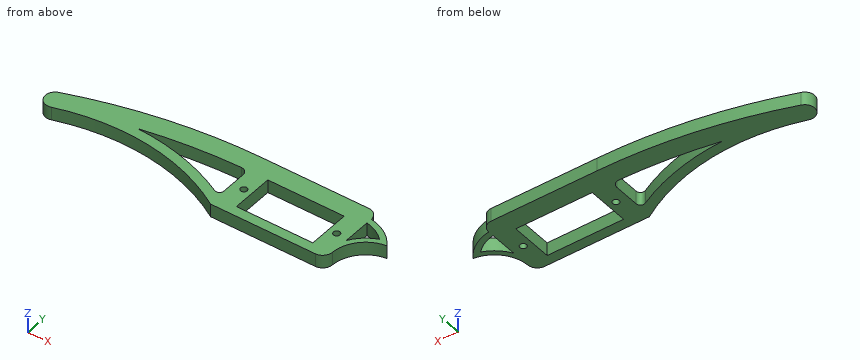
from build123d import *

# Parameters (mm, degrees)
SKETCH_R  = 1
SKETCH_W  = 23.3
SKETCH_H  = 12.8
PAD_DEPTH = 4


with BuildPart() as part:
    # Sketch → Pad (new body)
    with BuildSketch(Plane.XY):
        with BuildLine():
            Line((-17.65, 12.4), (14.65, 12.4))
            ThreePointArc((17.65, 9.4), (16.77132, 11.52132), (14.65, 12.4))
            ThreePointArc((26.84, 3.51), (22.883245, 7.450836), (17.65, 9.4))
            ThreePointArc((26.84, 3.51), (20.406481, 0.259943), (17.65, -6.4))
            ThreePointArc((14.65, -9.4), (16.77132, -8.52132), (17.65, -6.4))
            Line((14.65, -9.4), (-17.27, -9.4))
            ThreePointArc((-17.27, -9.4), (-43.226691, -0.259051), (-70.626477, -2.82))
            ThreePointArc((-72.67, 2.821276), (-74.470639, -1.021762), (-70.626477, -2.82))
            ThreePointArc((-17.65, 12.4), (-45.579054, 10.017677), (-72.67, 2.821276))
        make_face()
        with Locations((-14.15, 0)):
            Circle(SKETCH_R, mode=Mode.SUBTRACT)
        with Locations((14.15, 0)):
            Circle(SKETCH_R, mode=Mode.SUBTRACT)
        Rectangle(SKETCH_W, SKETCH_H, mode=Mode.SUBTRACT)
        with BuildLine():
            Line((17.65, 7.636176), (17.65, -0.84))
            ThreePointArc((23.88, 4.42), (20.301686, 2.338754), (17.65, -0.84))
            ThreePointArc((23.88, 4.42), (21.017458, 6.51712), (17.65, 7.636176))
        make_face(mode=Mode.SUBTRACT)
        with BuildLine():
            Line((-17.66615, -3.466269), (-17.66615, 4.388555))
            ThreePointArc((-17.66615, 4.388555), (-18.261027, 5.807615), (-19.69, 6.378267))
            ThreePointArc((-19.69, 6.378267), (-34.408413, 5.451456), (-48.98, 3.18))
            ThreePointArc((-19.59, -4.623545), (-33.83794, 0.961961), (-48.98, 3.18))
            ThreePointArc((-19.59, -4.623545), (-18.300889, -4.58882), (-17.66615, -3.466269))
        make_face(mode=Mode.SUBTRACT)
    extrude(amount=PAD_DEPTH)


solid = part.part
Geometry: final body of the model. Coordinates: model frame, mm. Round coordinates to 2 decimals unless told otherwise and drop trailing zeros. Loops run counter-clockwise (first coordinate to the right, second up) from the corner with the lowest first, then second, coordinate; pieces in that order, holes last. Notation, with made-up numbers: (-2.5, 5) -> (12.5, 5) arc R21 ccw to (12.5, 26) -> close; hole circle Ø10 at (-17, -23). An arc over 180 degrees is marked (long way). One line per question, with ' | ' between items. Start each with the question number.
1. Section D-D on y = -8. Output: boundary loops of the cut face in (x, z), and give its area (3 significant figures).
2. Section A-A on x = 10. Output: boundary loops of the cut face in (y, z).
3. Section C-C on x = -14.15. Output: boundary loops of the cut face in (y, z), and give its area (3 significant figures).
4. Line query: line 1 along Y through (x, z) = (14.15, 3.2); line 2 along Y through (x, z) = (-0.5, 0.95); line 3 along Y through (x, z) = (-54, 3.8). Output: solid intervals per line, ascending. Write a range as [from, to].
5. Contact query for flat-ended pins moving along their axis: pin 1 (2 mm diameter, centred on x = -50.5, z = 2, fed in from -Y); pin 2 (1.2 mm diameter, centred on y = -3, z = 2, fed in from +X); pin 3 (1 mm diameter, centred on y = -0.5, z = 1.5, fed in from -X); pin 4 (1.2 mm diameter, centred on y = -2.5, z = 1.5, fed in from -X). Output: stop coordinate, or through.
6. Section B-B on z = 2.3. Output: boundary loops of the cut face in (x, y), and give its area (3 significant figures).
Returned:
1) outline: (-19.64, 0) -> (17.19, 0) -> (17.19, 4) -> (-19.64, 4) -> close | area: 147 mm2
2) outline: (-9.4, 0) -> (-6.4, 0) -> (-6.4, 4) -> (-9.4, 4) -> close; (6.4, 0) -> (12.4, 0) -> (12.4, 4) -> (6.4, 4) -> close
3) outline: (-9.4, 0) -> (-1, 0) -> (-1, 4) -> (-9.4, 4) -> close; (1, 0) -> (12.4, 0) -> (12.4, 4) -> (1, 4) -> close | area: 79.2 mm2
4) line 1: y = [-9.4, -1], [1, 12.4] | line 2: y = [-9.4, -6.4], [6.4, 12.4] | line 3: y = [0.16, 8.32]
5) pin 1: stops at y = 0.2 | pin 2: stops at x = 18.62 | pin 3: stops at x = -74.65 | pin 4: stops at x = -73.97
6) outline: (-72.67, 2.82) arc R3 ccw to (-70.63, -2.82) arc R64.23 cw to (-17.27, -9.4) -> (14.65, -9.4) arc R3 ccw to (17.65, -6.4) arc R10.36 cw to (26.84, 3.51) arc R13.18 ccw to (17.65, 9.4) arc R3 ccw to (14.65, 12.4) -> (-17.65, 12.4) arc R160.79 ccw to start; hole (-48.98, 3.18) arc R67.22 cw to (-19.59, -4.62) arc R1.31 ccw to (-17.67, -3.47) -> (-17.67, 4.39) arc R1.99 ccw to (-19.69, 6.38) arc R160.79 ccw to start; hole circle Ø2 at (-14.15, 0); hole (-11.65, -6.4) -> (11.65, -6.4) -> (11.65, 6.4) -> (-11.65, 6.4) -> close; hole circle Ø2 at (14.15, 0); hole (17.65, -0.84) arc R11.93 cw to (23.88, 4.42) arc R11.44 ccw to (17.65, 7.64) -> close | area: 967 mm2
